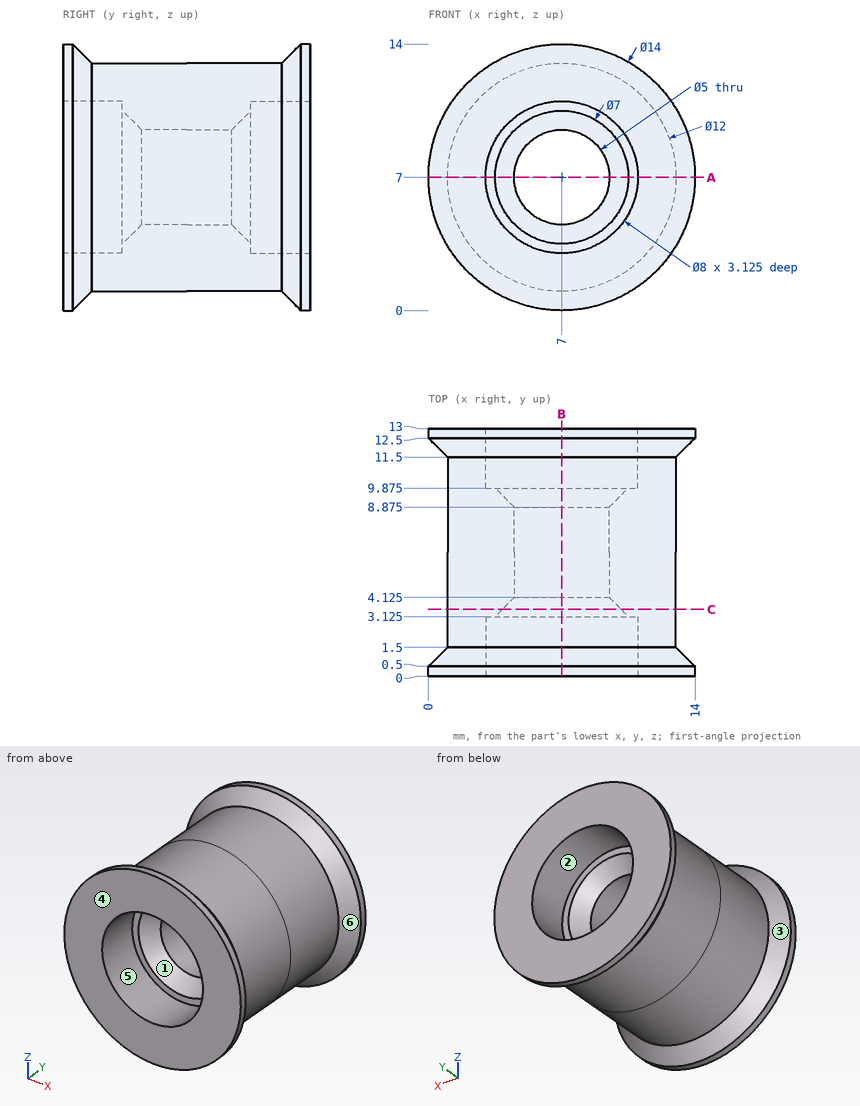
Geometry check sheet. Reference: drawing and pictorial views, mm from the part's lowest x, y, z. A direction names the side the tool comes from. Round coordinates to 2 decimals unless told otherwise and drop trailing zeros. Loops run counter-clockwise (first coordinate to the right, second up) from the corner with the lowest first, then second, coordinate; pieces in that order, holes last. Notation, with made-up numbers: (63, -23) -> (87, -23) arc R17 cw to (87, -10) -> close; hole circle Ø11 at (30.25, 87.25). An arc over 180 degrees is marked (long way). Answer as a JSON object with one key per item and string values. Group by question number.
Item 1: Cross-section at C-C, the plane y = 3.5. Record the cut outline in (x, z) (3 decimals).
Item 2: Set-up check for the marked faces 1, 2 and 3: record each of +Z, -Z, +X, -X, +Y, -Y from which the full face is reachable in a straight line by a thin tool's end or side.
Item 3: Cross-section at A-A, the plane z = 7. Record the cut outline in (x, y) (3 decimals), plus the area to 4 significant figures.
Item 4: Depth check by flat-ended pin: pin 1 Ø4 at (y, z) = (4, 1.5) entering from -X; pin 2 Ø6 at (y, z) = (9, 11.5) entering from -X; pin 3 Ø5 at (x, y) = (4, 1.5) entering from +Z. Enter the tip coordinate at first touch or a pass-through.
Item 5: Thickness scan on line 1 along Z through (x, y) = (7, 5.25); line 2 along Z through (x, y) = (7, 11.2). Record the ranges inside material, lowest first.
Item 6: Cross-section at B-B, the plane x = 7. Record the cut outline in (y, z) (3 decimals).
Item 7: Release check for a two-part mould opening along X. For the marked faces 4, 5 and 6 record: pulls with the +X half, pulls with the -X half, needs draft (parallel to the pull), parting line crosses it, or undercut.
Determined:
{
 "1": {"outline": "circle Ø12 at (7, 7); hole circle Ø6.25 at (7, 7)"},
 "2": {"face 1": "-Y", "face 2": "+Y", "face 3": "none"},
 "3": {"outline": "(0, 0) -> (3, 0) -> (3, 3.125) -> (3.5, 3.125) -> (4.5, 4.125) -> (4.5, 8.875) -> (3.5, 9.875) -> (3, 9.875) -> (3, 13) -> (0, 13) -> (0, 12.5) -> (1, 11.5) -> (1, 1.5) -> (0, 0.5) -> close; (9.5, 4.125) -> (10.5, 3.125) -> (11, 3.125) -> (11, 0) -> (14, 0) -> (14, 0.5) -> (13, 1.5) -> (13, 11.5) -> (14, 12.5) -> (14, 13) -> (11, 13) -> (11, 9.875) -> (10.5, 9.875) -> (9.5, 8.875) -> close", "area": "74.25 mm²"},
 "4": {"pin 1": "stops at x = 2.13", "pin 2": "stops at x = 1.19", "pin 3": "stops at z = 13.96"},
 "5": {"line 1": "z = 1 to 4.5, 9.5 to 13", "line 2": "z = 1 to 3, 11 to 13"},
 "6": {"outline": "(0, 0) -> (0.5, 0) -> (1.5, 1) -> (11.5, 1) -> (12.5, 0) -> (13, 0) -> (13, 3) -> (9.875, 3) -> (9.875, 3.5) -> (8.875, 4.5) -> (4.125, 4.5) -> (3.125, 3.5) -> (3.125, 3) -> (0, 3) -> close; (0, 11) -> (3.125, 11) -> (3.125, 10.5) -> (4.125, 9.5) -> (8.875, 9.5) -> (9.875, 10.5) -> (9.875, 11) -> (13, 11) -> (13, 14) -> (12.5, 14) -> (11.5, 13) -> (1.5, 13) -> (0.5, 14) -> (0, 14) -> close"},
 "7": {"face 4": "needs draft", "face 5": "undercut", "face 6": "parting line crosses it"}
}
